Autodesk Inventor part; units mm, degrees
ref_plane "YZ Plane" through (0, 0, 0) normal (1, 0, 0) x (0, 1, 0)
ref_plane "XZ Plane" through (0, 0, 0) normal (0, 1, 0) x (-1, 0, 0)
ref_plane "XY Plane" through (0, 0, 0) normal (0, 0, 1) x (1, 0, 0)
sketch "Sketch1" plane through (0, 0, 0) normal (0, 0, 1) x (1, 0, 0)
  circle A0 centre (0, 0) radius 6.35
  dimension "d0" = 12.7
extrude "Extrusion1" add sketch "Sketch1" along normal blind 1.5875
sketch "Sketch2" plane through (0, 0, 1.5875) normal (0, 0, 1) x (1, 0, 0)
  circle A0 centre (0, 0) radius 6.35
  circle A1 centre (0, 0) radius 3.9688
  dimension "d3" = 7.9375
extrude "Extrusion2" add sketch "Sketch2" along normal blind 27.3495 contours A1
fillet "Fillet1" radius 3.175 1 edges at (-3.9688, 0, 1.5875)
sketch "Sketch3" plane through (0, 0, 28.937) normal (0, 0, 1) x (1, 0, 0)
  circle A0 centre (0, 0) radius 3.9687
hole "Hole1" at (0, 0, 28.937) direction (0, 0, -1) diameter 4.9784 end through all
properties part number "Pneumatic Standoff Curved" material "Aluminum 6061"
Can you work these out from the model? Positions are in its coordinate system, mm. A direction names the side the tool comes from. Round coordinates to 2 decimals unless told otherwise and drop trailing zeros. Loops run counter-clockwise (first coordinate to the right, second up) from the corner with the lowest first, then second, coordinate; pieces in that order, holes last. Notation, with made-up numbers: (-24, -0.75) - (15, -0.75) arc R23 cw to (15, 22.25) - close; hole circle Ø5 at (24, -21.5). An arc over 180 degrees is marked (long way). Write item = value, one per line. Start each with the question number.
(1) For P1, Ø4, axis at y = -5, z = 14, coming from the +X side; P2, Ø5, axis at x = -3, z = 16.5, coming from the +Y side, each with a flat end and sliding along its axis, tell me the tip position at first contact or that it passes through.
(2) If we section it at D-D (z = 2.5): Please give me the cut outline in (x, y).
(3) If we mould it in two halves opening along X, with no side actions, what happens to faces 1 (the face through (-1.38, 6.2, 0.78)), 2 (the face through (3, 0, 0)), 3 (the face through (-0.748, -2.374, 14.266))? For each: released by +X, released by -X, zero draft, split by the parting line, or undercut.
(4) For faces 4 (the face through (3.666, 1.52, 16.629)), 5 (the face through (2, 2, 28.937)), which set-ups out of +Z, -Z, +X, -X, +Y, -Y let a thin tool reach every point of the face, with its end or its side?
(5) If we section it at C-C (z = 11.75): Please give me the cut outline in (x, y), and give its area (3 significant figures).
(6) If I drill on probe 1 along Y at (x, z) = (0, 9.5); probe 2 along X at (y, z) = (1, 15); probe 3 along Y at (x, z) = (-0.5, 11), over which ranges is the centre line in solid material (lowest first)? Write a range as [from, to].
Ans:
q1.P1 = 2.6
q1.P2 = 3.94
q2.outline = circle Ø9.64 at (0, 0); hole circle Ø4.98 at (0, 0)
q3.face_1 = split by the parting line
q3.face_2 = zero draft
q3.face_3 = undercut
q4.face_4 = +Z
q4.face_5 = +Z, +X, -X, +Y, -Y
q5.outline = circle Ø7.94 at (0, 0); hole circle Ø4.98 at (0, 0)
q5.area = 30.0 mm²
q6.probe_1 = [-3.97, -2.49], [2.49, 3.97]
q6.probe_2 = [-3.84, -2.28], [2.28, 3.84]
q6.probe_3 = [-3.94, -2.44], [2.44, 3.94]
